Here's how the part is built. I have some questions about the finished solid (model axes, mm). A direction names the side the tool comes from. Coordinates: 2 decimals unless noted, no trailing zeros. Loops run counter-clockwise (first coordinate to the right, second up) from the corner with the lowest first, then second, coordinate; pieces in that order, holes last. Notation, with made-up numbers: (89, 46.5) -> (126, 46.5) arc R12 ccw to (126, 60.5) -> close; hole circle Ø7 at (5.25, -31). An arc over 180 degrees is marked (long way). Answer as a JSON object with one key per item and string values. Group by question number.
Q1. I'm going to push flat-ended pins straight in: pin 1 (0.9 mm diameter, centred on x = 4.5, y = 0.5, fed in from +Z); pin 2 (2 mm diameter, centred on x = 3.5, z = 1, fed in from +Y); pin 3 (0.8 mm diameter, centred on x = 3.5, z = 0, fed in from -Y). Where does each tip first touch, or does it pass through?
Q2. I want a section at C-C on x = -1. Write out the boundary of the cut face in (y, z).
Q3. Thinking about a two-plate mould opening in X: for faces 6 (the flat face through (3.5, 0.5, 0)), 7 (the flat face through (1.5, 4, 0)), 8 (the flat face through (0, 0, 0)), 9 (the flat face through (-1.5, 4, 0)), which applies, released by +X, released by -X, zero draft, split by the parting line, or undercut?
Q4. I want a section at D-D on y = 2.85. Write out the boundary of the cut face in (x, z), then the cut area to 3 significant figures.
Q5. I want a section at B-B on y = 4.05. Write out the boundary of the cut face in (x, z).
Q6. I need wall thicknesses on line 1 (Y direction, x = -3.25, z = 0.15); line 2 (Y direction, x = -2.25, z = 0.9); line 3 (X direction, y = 0.75, z = 0.95). Which ranges of each line are inside material? Lowest first, please.
Q7. On a 3-axis mill with a long thin cutter (end or side, diameter ignored), from which of +Z, -Z, +X, -X, +Y, -Y can I reach the whole of each face in a straight line? I mean faces 1 (the flat face through (0, 4, 0.76)), 2 (the flat face through (3.5, 0.8, 0)), 3 (the flat face through (0, 4, -0.76)), 4 (the flat face through (-3.5, 0.8, 0)), 5 (the flat face through (0, 3.5, -1.2)). Say none if no direction works.
```python
from build123d import *

# Parameters (mm, degrees)
SKETCH1_W           = 6
SKETCH1_H           = 3.5
BOSS_EXTRUDE1_DEPTH = 3.5
FILLET1_R           = 0.2
SKETCH2_W           = 3
SKETCH2_H           = 1.52
BOSS_EXTRUDE2_DEPTH = 1.07
FILLET2_R           = 0.1
SKETCH3_W           = 1
SKETCH3_H           = 0.3
CIRPATTERN1_COUNT   = 2


with BuildPart() as part:
    # Sketch1 → Boss-Extrude1 (new body)
    with BuildSketch(Plane(origin=(0, 0, 0), x_dir=(1, 0, 0), z_dir=(0, 1, 0))):
        Rectangle(SKETCH1_W, SKETCH1_H)
    extrude(amount=BOSS_EXTRUDE1_DEPTH)

    # Fillet1
    fillet1_edges = [part.edges().sort_by_distance(p)[0] for p in [
        (-3, 1.75, -1.75),
        (3, 1.75, -1.75),
        (3, 1.75, 1.75),
        (-3, 1.75, 1.75),
    ]]
    fillet(fillet1_edges, radius=FILLET1_R)

    # Sketch2 → Boss-Extrude2 (add)
    with BuildSketch(Plane(origin=(0, 3.5, 0), x_dir=(1, 0, 0), z_dir=(0, 1, 0))):
        Rectangle(SKETCH2_W, SKETCH2_H)
    extrude(amount=BOSS_EXTRUDE2_DEPTH)

    # Fillet2
    fillet2_edges = [part.edges().sort_by_distance(p)[0] for p in [
        (1.5, 3.5, 0),
        (1.5, 4.035, 0.76),
        (0, 3.5, -0.76),
        (1.5, 4.035, -0.76),
        (-1.5, 3.5, 0),
        (-1.5, 4.035, -0.76),
        (0, 3.5, 0.76),
        (-1.5, 4.035, 0.76),
        (1.5, 4.57, 0),
        (0, 4.57, -0.76),
        (-1.5, 4.57, 0),
        (0, 4.57, 0.76),
    ]]
    fillet(fillet2_edges, radius=FILLET2_R)

    # Sweep1: sweep along a path in Sketch4
    with BuildLine(Plane.XY) as sweep1_path:
        Line((3, 0.65), (4.02, 0.65))
        ThreePointArc((4.02, 0.65), (4.196776695, 0.576776695), (4.27, 0.4))
        ThreePointArc((4.27, 0.4), (4.343223305, 0.223223305), (4.52, 0.15))
        Line((4.52, 0.15), (5.27, 0.15))
    # Sketch3 → Sweep1 (sweep)
    with BuildSketch(Plane(origin=(3, 0, 0), x_dir=(0, 0, -1), z_dir=(1, 0, 0))):
        with Locations((0, 0.65)):
            Rectangle(SKETCH3_W, SKETCH3_H)
    sweep1 = sweep(path=sweep1_path.line)

    # CirPattern1: Sweep1 ×2 about axis
    cirpattern1_axis = Axis((0, 4.7985, 0), (0, -1, 0))
    for i in range(1, CIRPATTERN1_COUNT):
        add(sweep1.rotate(cirpattern1_axis, i * 360 / CIRPATTERN1_COUNT))


solid = part.part
```
Result set:
{
 "1": {"pin 1": "stops at z = 0.5", "pin 2": "stops at y = 3.5", "pin 3": "stops at y = 0.5"},
 "2": {"outline": "(0, -1.75) -> (3.5, -1.75) -> (3.5, -0.86) arc R0.1 cw to (3.6, -0.76) -> (4.47, -0.76) arc R0.1 ccw to (4.57, -0.66) -> (4.57, 0.66) arc R0.1 ccw to (4.47, 0.76) -> (3.6, 0.76) arc R0.1 cw to (3.5, 0.86) -> (3.5, 1.75) -> (0, 1.75) -> close"},
 "3": {"face 6": "undercut", "face 7": "released by +X", "face 8": "zero draft", "face 9": "released by -X"},
 "4": {"outline": "(-3, -1.55) arc R0.2 ccw to (-2.8, -1.75) -> (2.8, -1.75) arc R0.2 ccw to (3, -1.55) -> (3, 1.55) arc R0.2 ccw to (2.8, 1.75) -> (-2.8, 1.75) arc R0.2 ccw to (-3, 1.55) -> close", "area": "21.0 mm²"},
 "5": {"outline": "(-1.5, -0.66) arc R0.1 ccw to (-1.4, -0.76) -> (1.4, -0.76) arc R0.1 ccw to (1.5, -0.66) -> (1.5, 0.66) arc R0.1 ccw to (1.4, 0.76) -> (-1.4, 0.76) arc R0.1 ccw to (-1.5, 0.66) -> close"},
 "6": {"line 1": "y = 0.5 to 0.8", "line 2": "y = 0 to 3.5", "line 3": "x = -3 to 3"},
 "7": {"face 1": "+Z, +X, -X, +Y", "face 2": "+Z, -Z, +X, +Y", "face 3": "-Z, +X, -X, +Y", "face 4": "+Z, -Z, -X, +Y", "face 5": "+Y"}
}
